from build123d import *

# Parameters (mm, degrees)
F1_DEPTH    = 3
F2_DEPTH    = 0.25
F3_DEPTH    = 0.25
F4_R        = 2
F5_R        = 1.5
F6_R        = 5
F7_T1_DEPTH = 40.5120657328


# Not quite as in the source:
# - a fillet or chamfer that OpenCascade refuses, or shapes differently, is made with other operations: its cross-section is extruded or revolved along the edge and cut away or added


with BuildPart() as f1:
    # F0 (on Front) → F1 (new body)
    with BuildSketch(Plane.XZ):
        with BuildLine():
            ThreePointArc((3.6544098407, -9.5319570974), (-8.5955901593, -21.7819570974), (-20.8455901593, -9.5319570974))
            Line((-20.8455901593, -9.5319570974), (-20.8455901593, 12.4680429026))
            Line((-20.8455901593, 12.4680429026), (-23.8455901593, 12.4680429026))
            Line((-23.8455901593, 12.4680429026), (-23.8455901593, -9.5319570974))
            Line((-23.8455901593, -9.5319570974), (-23.8455901593, -21.7819570974))
            Line((-23.8455901593, -21.7819570974), (-28.5955901593, -26.7819570974))
            Line((-28.5955901593, -26.7819570974), (-8.5955901593, -26.7819570974))
            Line((-8.5955901593, -26.7819570974), (11.4044098407, -26.7819570974))
            Line((11.4044098407, -26.7819570974), (6.6544098407, -21.7819570974))
            Line((6.6544098407, -21.7819570974), (6.6544098407, 12.4680429026))
            Line((6.6544098407, 12.4680429026), (3.6544098407, 12.4680429026))
            Line((3.6544098407, 12.4680429026), (3.6544098407, -9.5319570974))
        make_face()
    extrude(amount=F1_DEPTH)

    # F2 (add): a face of the model
    f2_faces = [f1.faces().sort_by_distance(p)[0] for p in [
        (-20.8455901593, -1.5, 1.4680429026),
    ]]
    extrude(f2_faces, amount=F2_DEPTH)

    # F3 (add): a face of the model
    f3_faces = [f1.faces().sort_by_distance(p)[0] for p in [
        (3.6544098407, -1.5, 1.4680429026),
    ]]
    extrude(f3_faces, amount=F3_DEPTH)

    # F4
    f4_edges = [f1.edges().sort_by_distance(p)[0] for p in [
        (-8.59559, 0, -21.781957),
    ]]
    fillet(f4_edges, radius=F4_R)

    # F5
    f5_edges = [f1.edges().sort_by_distance(p)[0] for p in [
        (11.40441, -1.5, -26.781957),
        (-28.59559, -1.5, -26.781957),
    ]]
    fillet(f5_edges, radius=F5_R)

    # F6
    f6_edges = [f1.edges().sort_by_distance(p)[0] for p in [
        (-23.84559, -1.5, -21.781957),
        (6.65441, -1.5, -21.781957),
    ]]
    fillet(f6_edges, radius=F6_R)

    # F7: fillet of radius 1.5 on 1 edges, made by hand

    # F7_s2 → F7_t1 (cut)
    with BuildSketch(Plane.YZ.offset(-28.8516230257)):
        with BuildLine():
            ThreePointArc((-3, -25.2819570974), (-2.5606601718, -26.3426172691), (-1.5, -26.7819570974))
            Line((-1.5, -26.7819570974), (-3, -26.7819570974))
            Line((-3, -26.7819570974), (-3, -25.2819570974))
        make_face()
    extrude(amount=F7_T1_DEPTH, mode=Mode.SUBTRACT)


solid = f1.part
Part model, mm, in its own coordinate system. A direction names the side the tool comes from. Round coordinates to 2 decimals unless told otherwise and drop trailing zeros. Write each loop counter-clockwise with the first axis right and the second up, starting at its lowest first coordinate (ties: lowest second). Pieces come first, ordered by that corner, then holes. Notation, with made-up numbers: M 78.5,41 L 112.5,41 A18 cw 112.5,62 Z; hole C 11,75 d7. An arc over 180 degrees is marked long. Return JSON: item names as keys, results as strings. Group by question number.
(1) Which spindle directions (+Z, -Z, +X, -X, +Y, -Y) get a long thin tool onto all of the face, cutting with end or side? Do faces 1 (the face through (6.654, -1, -4)), 2 (the face through (3.8, -0.9, -9.532)), 3 (the face through (3.404, -1, 2)). Say none if no direction does.
(2) Pin check, flat tips, straight feed: pin 1 Ø1.5 at (y, z) = (-1.5, -9) entering from -X; pin 2 Ø8 at (x, z) = (1, -3.5) entering from +Y; pin 3 Ø1.5 at (y, z) = (-2, 1.5) entering from +X. Stop position of each tip, or through.
(3) Saw through at A-A on z = -6.5. Write the cut outline in (x, y).
(4) Two-plate mould, pull along Z, no slides. Class faces 4 (the face through (5, -1, 12.468)), 5 (the face through (-20.976, -0.937, -9.532)), 6 (the face through (-6, -3, -22)): +Z half, -Z half, draft (parallel to the pull), parting line (faces both ways), or undercut.
(5) Drill centre lines: probe 1 along X at (y, z) = (-1.15, 6.5); probe 2 along X at (y, z) = (-2.9, -20.5); probe 3 along Z at (x, y) = (-1.5, -1.1). Where is each one in solid material? Low to high.
Returned:
{
 "1": {"face 1": "+Z, +X, +Y, -Y", "face 2": "+Y", "face 3": "+Z, +Y, -Y"},
 "2": {"pin 1": "x = -23.85", "pin 2": "y = 0", "pin 3": "x = 6.65"},
 "3": {"outline": "M -23.85,-3 L -20.6,-3 L -20.6,0 L -23.85,0 Z; M 3.4,-3 L 6.65,-3 L 6.65,0 L 3.4,0 Z"},
 "4": {"face 4": "+Z half", "face 5": "undercut", "face 6": "draft"},
 "5": {"probe 1": "-23.85 to -20.6, 3.4 to 6.65", "probe 2": "-23.9 to -14.05, -3.14 to 6.71", "probe 3": "-26.78 to -19.78"}
}
